Here's how the part is built. I have some questions about the finished solid (model axes, mm). A direction names the side the tool comes from. Round coordinates to 2 decimals unless told otherwise and drop trailing zeros. Write each loop counter-clockwise with the first axis right and the second up, starting at its lowest first coordinate (ties: lowest second). Pieces come first, ordered by that corner, then holes. Notation, with made-up numbers: (25.25, -32) -> (80.25, -32) arc R31 cw to (80.25, 2) -> close; hole circle Ø9 at (31, 54). An arc over 180 degrees is marked (long way). Answer as CSV lines item,"result".
```python
from build123d import *

# Parameters (mm, degrees)
SKETCH1_R           = 92.5
SKETCH1_R_2         = 90
BOSS_EXTRUDE1_DEPTH = 90
SKETCH2_R           = 100
SKETCH2_R_2         = 90
BOSS_EXTRUDE2_DEPTH = 3
MIRROR1_START       = 93
MIRROR1_OUTLINE_R   = 92.5
MIRROR1_OUTLINE_R_2 = 90
MIRROR1_DEPTH       = 87


# Read off the part's stored shape, not the designer's step: Mirror1
with BuildPart() as part:
    # Sketch1 → Boss-Extrude1 (new body)
    with BuildSketch(Plane(origin=(0, 0, 0), x_dir=(1, 0, 0), z_dir=(0, 1, 0))):
        with Locations(Location((0, 0, 0), (0, 0, 90))):
            Circle(SKETCH1_R)
        with Locations(Location((0, 0, 0), (0, 0, 90))):
            Circle(SKETCH1_R_2, mode=Mode.SUBTRACT)
    extrude(amount=BOSS_EXTRUDE1_DEPTH)

    # Sketch2 → Boss-Extrude2 (add)
    with BuildSketch(Plane(origin=(0, 90, 0), x_dir=(1, 0, 0), z_dir=(0, 1, 0))):
        with Locations(Location((0, 0, 0), (0, 0, 270))):
            Circle(SKETCH2_R)
        with Locations(Location((0, 0, 0), (0, 0, 90))):
            Circle(SKETCH2_R_2, mode=Mode.SUBTRACT)
    extrude(amount=BOSS_EXTRUDE2_DEPTH)

    # Mirror1 outline → Mirror1 (add)
    with BuildSketch(Plane(origin=(0, 0, 0), x_dir=(1, 0, 0), z_dir=(0, 1, 0)).offset(MIRROR1_START)):
        Circle(MIRROR1_OUTLINE_R)
        Circle(MIRROR1_OUTLINE_R_2, mode=Mode.SUBTRACT)
    extrude(amount=MIRROR1_DEPTH)


solid = part.part
```
1. If I drill on line 1 (X direction, y = 63, z = 0); line 2 (Y direction, x = 84.5, z = 53), over which ranges is the centre line in solid material (lowest first)?
Numbers:
line 1,"x = -92.5 to -90, 90 to 92.5"
line 2,"y = 90 to 93"
2. On a 3-axis mill with a long thin cutter (end or side, diameter ignored), from which of +Z, -Z, +X, -X, +Y, -Y can I reach the whole of each face in a straight line? I mean faces 1 (the face through (-88, 93, 29)), 2 (the face through (20, 180, 89)), 3 (the face through (90.3, 44.37, 20.05)). Say none if no direction works.
Numbers:
face 1,"+Y"
face 2,"+Z, -Z, +X, -X, +Y"
face 3,"-Y"
3. Suppose I cut it at A-A on z = 0. Please give me the cut outline in (x, y).
Numbers:
outline,"(-100, 90) -> (-92.5, 90) -> (-92.5, 0) -> (-90, 0) -> (-90, 180) -> (-92.5, 180) -> (-92.5, 93) -> (-100, 93) -> close; (90, 0) -> (92.5, 0) -> (92.5, 90) -> (100, 90) -> (100, 93) -> (92.5, 93) -> (92.5, 180) -> (90, 180) -> close"
4. Suppose I cut it at B-B on x = 80. Please give me the cut outline in (y, z), and give its area (3 significant figures).
Numbers:
outline,"(0, -46.44) -> (90, -46.44) -> (90, -60) -> (93, -60) -> (93, -46.44) -> (180, -46.44) -> (180, -41.23) -> (0, -41.23) -> close; (0, 41.23) -> (180, 41.23) -> (180, 46.44) -> (93, 46.44) -> (93, 60) -> (90, 60) -> (90, 46.44) -> (0, 46.44) -> close"
area,"1,950 mm^2"
5. For pin 1 Ø5 at (y, z) = (74.5, 31.5) entering from +X; pin 2 Ø1 at (x, y) = (48, 60) entering from +Z; pin 3 Ø8 at (y, z) = (123.5, 56) entering from +X, each with a flat end and sliding along its axis, tell me the tip position at first contact or that it passes through.
Numbers:
pin 1,"stops at x = 87.84"
pin 2,"stops at z = 79.37"
pin 3,"stops at x = 76.5"
6. Suppose I cut it at C-C on y = 104. Please give me the cut outline in (x, z).
Numbers:
outline,"circle Ø185 at (0, 0); hole circle Ø180 at (0, 0)"
